Design review of the part shown in the three views and the two pictorial views. Dimensions are in mm from the part's minimum x, y and z. A direction names the side the tool comes from. Round coordinates to 2 decimals unless told otherwise and drop trailing zeros. Loops run counter-clockwise (first coordinate to the right, second up) from the corner with the lowest first, then second, coordinate; pieces in that order, holes last. Notation, with made-up numbers: (18, 7.25) -> (61, 7.25) arc R10 cw to (61, 18.25) -> close; hole circle Ø1 at (20, 3.25). An arc over 180 degrees is marked (long way). Use a Markdown table: item, result. Add a question column.
1) Consider section B-B on y = 7.5. Give the boundary of the cut face in (x, z), plus the area to 3 significant figures.
2) Consider section A-A on x = 5. Give the boundary of the cut face in (y, z).
3) Wall thickness on probe 1 along Z at (x, y) = (4.5, 13); probe 2 along Y at (x, z) = (5, 3.75); probe 3 along X at (y, z) = (5, 7.75): over which ranges is each line inside the solid? List them lowest first.
4) Mouldability with a two-part tool opening along Y and no side actions: class the marked faces 1, 2 and 3 as released by +Y, released by -Y, zero draft, split by the parting line, or undercut.
5) Insertion check: pin 1 (2 mm diameter, centred on y = 5.5, z = 7.5, fed in from -X); pin 2 (6 mm diameter, centred on x = 10.5, y = 1.5, fed in from -Z). Each pin has a flat end and moves straight along its axis. Give the tip position at first contact, or say it passes through.
6) Consider section D-D on z = 2.5. Give the boundary of the cut face in (x, y), plus the area to 3 significant figures.
7) Consider section C-C on x = 9. Give the boundary of the cut face in (y, z).
8) For the marked faces 4 and 5, list the 3-axis set-ups (+Z, -Z, +X, -X, +Y, -Y) from which the entire face can be reached by the end or side of a thin tool; tool diameter is ignored.
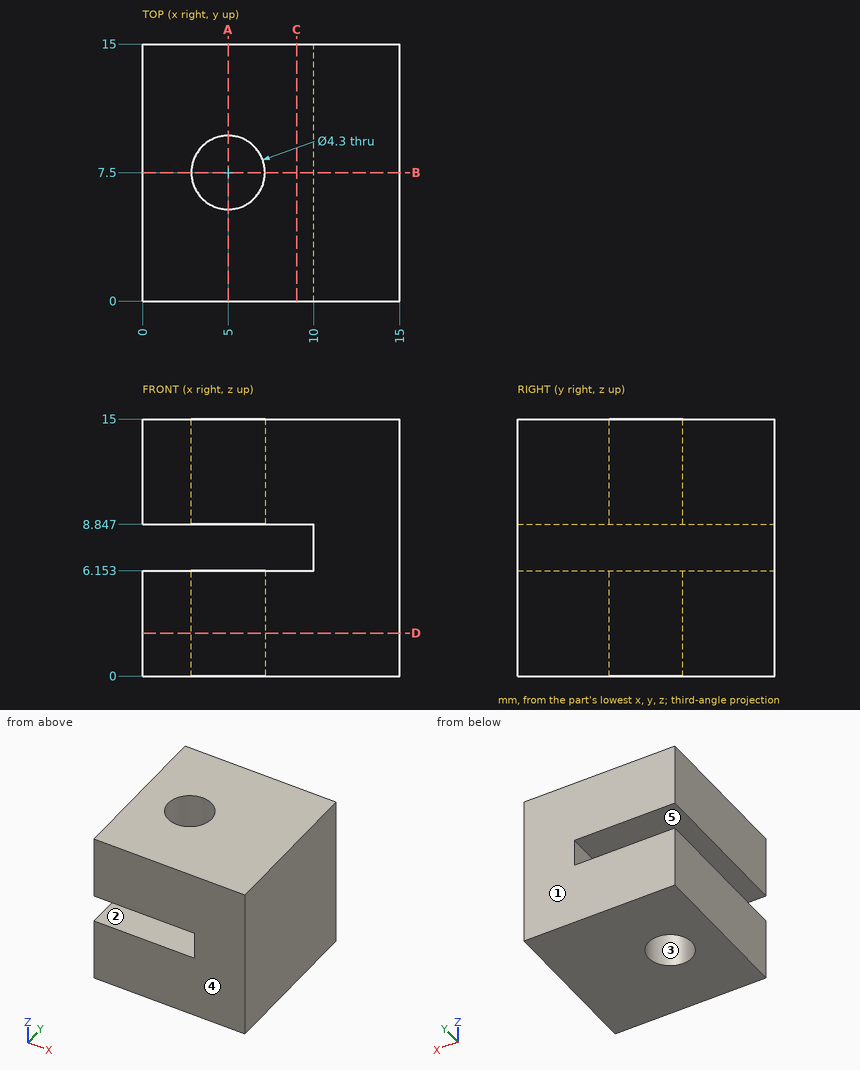
Result set:
| question | item | result |
|---|---|---|
| 1 | outline | (0, 0) -> (2.85, 0) -> (2.85, 6.15) -> (0, 6.15) -> close; (0, 8.85) -> (2.85, 8.85) -> (2.85, 15) -> (0, 15) -> close; (7.15, 0) -> (15, 0) -> (15, 15) -> (7.15, 15) -> (7.15, 8.85) -> (10, 8.85) -> (10, 6.15) -> (7.15, 6.15) -> close |
| 1 | area | 145 mm2 |
| 2 | outline | (0, 0) -> (5.35, 0) -> (5.35, 6.15) -> (0, 6.15) -> close; (0, 8.85) -> (5.35, 8.85) -> (5.35, 15) -> (0, 15) -> close; (9.65, 0) -> (15, 0) -> (15, 6.15) -> (9.65, 6.15) -> close; (9.65, 8.85) -> (15, 8.85) -> (15, 15) -> (9.65, 15) -> close |
| 3 | probe 1 | 0 to 6.15, 8.85 to 15 |
| 3 | probe 2 | 0 to 5.35, 9.65 to 15 |
| 3 | probe 3 | 10 to 15 |
| 4 | face 1 | released by +Y |
| 4 | face 2 | zero draft |
| 4 | face 3 | undercut |
| 5 | pin 1 | x = 10 |
| 5 | pin 2 | z = 0 |
| 6 | outline | (0, 0) -> (15, 0) -> (15, 15) -> (0, 15) -> close; hole circle Ø4.3 at (5, 7.5) |
| 6 | area | 210 mm2 |
| 7 | outline | (0, 0) -> (15, 0) -> (15, 6.15) -> (0, 6.15) -> close; (0, 8.85) -> (15, 8.85) -> (15, 15) -> (0, 15) -> close |
| 8 | face 4 | +Z, -Z, +X, -X, -Y |
| 8 | face 5 | -X, +Y, -Y |
